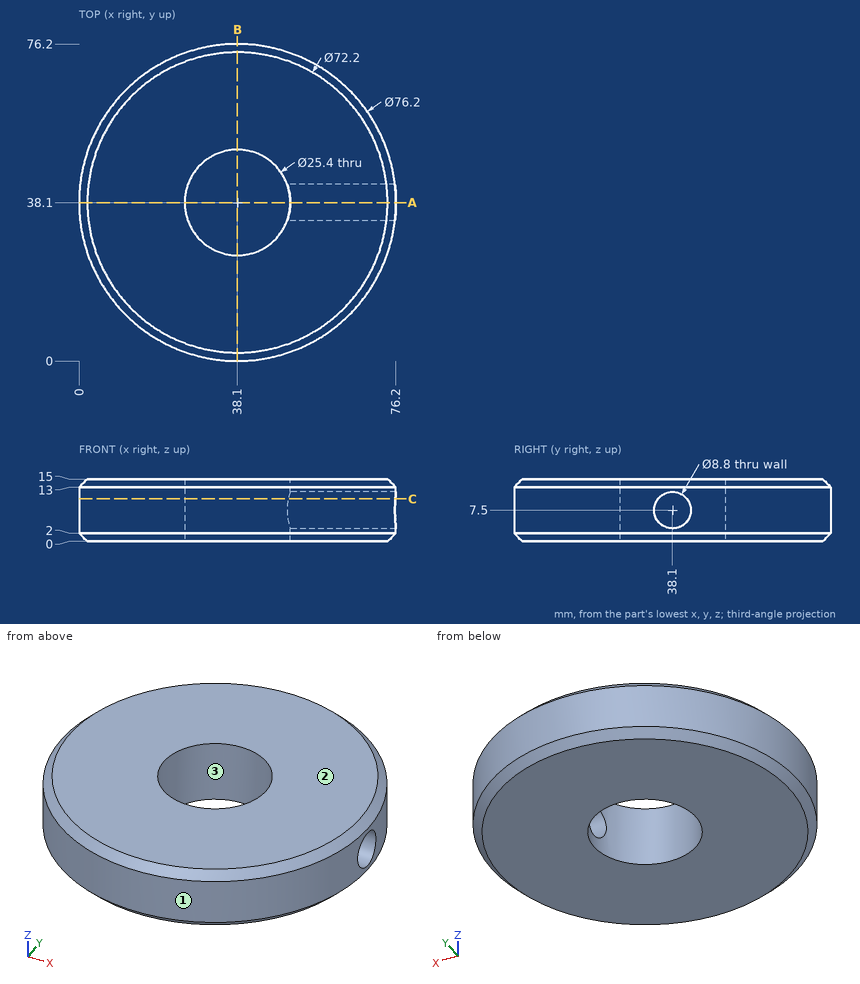
Geometry check sheet. Reference: drawing and pictorial views, mm from the part's lowest x, y, z. Round coordinates to 2 decimals unless told otherwise and drop trailing zeros. Write each loop counter-clockwise with the first axis right and the second up, starting at its lowest first coordinate (ties: lowest second). Pieces come first, ordered by that corner, then holes. Notation, with made-up numbers: (-21.75, 4) -> (7.25, 4) arc R28 ccw to (7.25, 23) -> close; hole circle Ø10 at (30.25, 77.25). An arc over 180 degrees is marked (long way). Put each result on its own line as item: value.
1) Depth check by flat-ended pin: P1, Ø8, axis at x = 63, y = 66.5, coming from the -Z side; P2, Ø1, axis at y = 26, z = 8.5, coming from the +X side; P3, Ø4, axis at x = 52.5, z = 11.5, coming from the +Y side; P4, Ø3, axis at x = 30, z = 9, coming from the -Y side. Enter the tip coordinate at first touch or a pass-through.
Recorded:
P1: stops at z = 0
P2: stops at x = 74.39
P3: stops at y = 74.13
P4: stops at y = 0.58
2) Release check for a two-part mould opening along X. For the marked faces 1, 2 and 3 record: pulls with the +X half, pulls with the -X half, needs draft (parallel to the pull), parting line crosses it, or undercut.
Recorded:
face 1: parting line crosses it
face 2: needs draft
face 3: undercut
3) Cross-section at C-C, the plane z = 10.25. Enter the section's corners in (x, y), plus the area to 3 significant figures.
Recorded:
outline: (50.33, 34.67) arc R12.7 cw (long way) to (50.33, 41.53) -> (76.04, 41.53) arc R38.1 ccw (long way) to (76.04, 34.67) -> close
area: 3,880 mm2
4) Cross-section at A-A, the plane y = 38.1. Enter the section's corners in (x, z).
Recorded:
outline: (0, 2) -> (2, 0) -> (25.4, 0) -> (25.4, 15) -> (2, 15) -> (0, 13) -> close; (50.8, 0) -> (74.2, 0) -> (76.2, 2) -> (76.2, 3.1) -> (50.8, 3.1) -> close; (50.8, 11.9) -> (76.2, 11.9) -> (76.2, 13) -> (74.2, 15) -> (50.8, 15) -> close
5) Cross-section at B-B, the plane x = 38.1. Enter the section's corners in (y, z), plus the area to 3 significant figures.
Recorded:
outline: (0, 2) -> (2, 0) -> (25.4, 0) -> (25.4, 15) -> (2, 15) -> (0, 13) -> close; (50.8, 0) -> (74.2, 0) -> (76.2, 2) -> (76.2, 13) -> (74.2, 15) -> (50.8, 15) -> close
area: 754 mm2
6) Thickness scan on probe 1 along Y at (x, z) = (38.1, 10.75); probe 2 along X at (y, z) = (32, 3.75); probe 3 along X at (y, z) = (45.5, 3.25). Record the ranges inside material, lowest first. Write a range as from..to.
Recorded:
probe 1: y = 0..25.4, 50.8..76.2
probe 2: x = 0.49..26.96, 49.24..75.71
probe 3: x = 0.73..27.78, 48.42..75.47
